```python
from build123d import *

# Parameters (mm, degrees)
BOSS_EXTRUDE1_DEPTH              = 5
F_97_0_0059_DIAMETER_HOLE1_D     = 1.600000102
F_97_0_0059_DIAMETER_HOLE1_DEPTH = 3
M2X0_4_TAPPED_HOLE1_D            = 1.6
M2X0_4_TAPPED_HOLE1_DEPTH        = 5.2
M2X0_4_TAPPED_HOLE1_TIP          = 0.480688495


with BuildPart() as part:
    # Sketch1 → Boss-Extrude1 (new body)
    with BuildSketch(Plane(origin=(0, 0, 0), x_dir=(1, 0, 0), z_dir=(0, 1, 0))):
        Polygon((0, 0), (2.25, 0), (2.25, 0.7), (9.75, 0.7), (9.75, 0), (12, 0), (12, 2.5), (0, 2.5), align=None)
    extrude(amount=BOSS_EXTRUDE1_DEPTH)

    # #97 (0.0059) Diameter Hole1
    with Locations(Plane(origin=(0, 0, -2.5), x_dir=(-1, 0, 0), z_dir=(0, 0, -1))):
        with Locations((-10.875, 2.5)):
            f_97_0_0059_diameter_hole1 = Hole(F_97_0_0059_DIAMETER_HOLE1_D / 2, depth=F_97_0_0059_DIAMETER_HOLE1_DEPTH)

    # M2x0.4 Tapped Hole1
    with Locations(Plane(origin=(0, 0, -2.5), x_dir=(-1, 0, 0), z_dir=(0, 0, -1))):
        with Locations((-6, 2.5)):
            Hole(M2X0_4_TAPPED_HOLE1_D / 2, depth=M2X0_4_TAPPED_HOLE1_DEPTH)
            with Locations((0, 0, -(M2X0_4_TAPPED_HOLE1_DEPTH + M2X0_4_TAPPED_HOLE1_TIP / 2))):  # 118° drill point
                Cone(0, M2X0_4_TAPPED_HOLE1_D / 2, M2X0_4_TAPPED_HOLE1_TIP, mode=Mode.SUBTRACT)

    # Mirror1: #97 (0.0059) Diameter Hole1 across plane
    add(f_97_0_0059_diameter_hole1.mirror(Plane(origin=(6, 0, 0), x_dir=(0, 0, 1), z_dir=(1, 0, 0))), mode=Mode.SUBTRACT)


solid = part.part
```
Could you check a few things on this model? Use its own coordinates, in mm. Give positions to 0.01 mm unless a question says otherwise; leave off trailing zeros. Loops run counter-clockwise (first coordinate to the right, second up) from the corner with the lowest first, then second, coordinate; pieces in that order, holes last. Notation, with made-up numbers: (75.25, 51.25) - (87.25, 51.25) arc R35 ccw to (87.25, 89.25) - close; hole circle Ø6 at (85.5, 55.25). An arc over 180 degrees is marked (long way). Use one line per item in the form item = value.
1. I want a section at A-A (x = 6). Please give me the cut outline in (y, z).
Response values:
outline = (0, -2.5) - (1.7, -2.5) - (1.7, -0.7) - (0, -0.7) - close; (3.3, -2.5) - (5, -2.5) - (5, -0.7) - (3.3, -0.7) - close
2. I want a section at D-D (y = 3.5). Please give me the cut outline in (x, z).
Response values:
outline = (0, -2.5) - (12, -2.5) - (12, 0) - (9.75, 0) - (9.75, -0.7) - (2.25, -0.7) - (2.25, 0) - (0, 0) - close
3. I want a section at C-C (y = 2.5). Please give me the cut outline in (x, z) (3 decimals), and give its area (3 significant figures).
Response values:
outline = (0, -2.5) - (0.325, -2.5) - (0.325, 0) - (0, 0) - close; (1.925, -2.5) - (5.2, -2.5) - (5.2, -0.7) - (2.25, -0.7) - (2.25, 0) - (1.925, 0) - close; (6.8, -2.5) - (10.075, -2.5) - (10.075, 0) - (9.75, 0) - (9.75, -0.7) - (6.8, -0.7) - close; (11.675, -2.5) - (12, -2.5) - (12, 0) - (11.675, 0) - close
area = 13.9 mm²
4. Thinking about a two-plate mould opening in Y: for faces 1 (the face through (5, 2, -0.7)), 2 (the face through (5.2, 2.5, -1.6)), 3 (the face through (6, 5, -1)), which applies, released by +Y, released by -Y, zero draft, split by the parting line, or undercut?
Response values:
face_1 = zero draft
face_2 = undercut
face_3 = released by +Y
5. I want a section at B-B (z = -1.25). Please give me the cut outline in (x, y) (3 decimals), and give its area (3 significant figures).
Response values:
outline = (0, 0) - (12, 0) - (12, 5) - (0, 5) - close; hole circle Ø1.6 at (1.125, 2.5); hole circle Ø1.6 at (6, 2.5); hole circle Ø1.6 at (10.875, 2.5)
area = 54.0 mm²
6. I'm going to push a flat-ended pin straight in: pin 1 Ø1.5 at (x, y) = (7.5, 3.5) entering from +Z. Where does the tip first touch, or does it pass through?
Response values:
pin_1 = -0.7
7. I need wall thicknesses on probe 1 along Y at (x, z) = (6, -1.55); probe 2 along X at (y, z) = (1.1, -0.25); probe 3 along Z at (x, y) = (3.25, 1.1). Which ranges of each line are inside material? Lowest first, please.
Response values:
probe_1 = 0 to 1.7, 3.3 to 5
probe_2 = 0 to 2.25, 9.75 to 12
probe_3 = -2.5 to -0.7
